Check sheet for the modelled part. Datum: model origin and axes. Units: mm. A direction names the side the tool comes from. Coordinates: 2 decimals unless noted, no trailing zeros. Write each loop counter-clockwise with the first axis right and the second up, starting at its lowest first coordinate (ties: lowest second). Pieces come first, ordered by that corner, then holes. Notation, with made-up numbers: M 49.5,-28.5 L 85.5,-28.5 A7 ccw 85.5,-24.5 Z; hole C -39,72.25 d9. An arc over 180 degrees is marked long. Answer as CSV lines item,"result". Start each with the question number.
1) Go/stop test with flat-tipped pins: pin 1 Ø3 at (y, z) = (-39.5, 29) entering from -X; pin 2 Ø3 at (x, z) = (-35.5, 78.5) entering from +Y; pin 3 Ø3 at (y, z) = (28.5, 2.5) entering from -X; pin 4 Ø12 at (x, y) = (-84.5, 26) entering from +Z. Record where each tip stops, or that it passes through.
2) Section check A-A (y = 28). Record the cut outline in (x, z) (3 decimals).
3) Material ranges on L1, parallel to Z at x = -96.5, y = -59.5 (3 decimals); L2, parallel to X at y = -33, z = 51.5 (3 decimals); L3, parallel to X at y = 55.5, z = 109, recorded low to high. Write a range as [from, to].
4) Section check B-B (x = -90). Record the cut outline in (y, z) (3 decimals).
5) Access from +Z, -Z, +X, -X, +Y, -Y to the whole of each face (thin tool, end or side, straight path). Record for faces 4 (the cylindrical face through (-64.831, -126.528, 57.817)), 5 (the flat face through (-76.2, 52, 110)), 6 (the flat face through (-9.525, 31, 58)).
6) Draft check along Z on faces 1 (the flat face through (-72, -21, 9.525)), 2 (the cylindrical face through (-107.2, -56.58, 109.6)), 3 (the flat face through (-67, -55, 0)). Enter one of: +Z half, -Z half, draft (parallel to the pull), parting line (faces both ways), or undercut.
from build123d import *

# Parameters (mm, degrees)
F1_DEPTH = 9.525
F2_DEPTH = 57.15


# Not quite as in the source:
# - ends of sketch curves that miss each other by under 0.0002 mm in the source are joined


with BuildPart() as f1:
    # F0 (on Top) → F1 (new body)
    with BuildSketch(Plane.XY):
        with BuildLine():
            Line((-9.525, -40.8894196153), (-9.525, 101.6))
            Line((-9.525, 101.6), (-76.2, 101.6))
            Line((-76.2, 101.6), (-76.2, 1.7757813176))
            ThreePointArc((-76.2, 1.7757813176), (-76.2737613091, -0.1585489984), (-76.4946168324, -2.0816447683))
            ThreePointArc((-76.4946168324, -2.0816447683), (-107.8980822653, -57.1580249287), (-168.0578880185, -77.1675992495))
            Line((-168.0578880185, -77.1675992495), (-168.0578880185, -143.8425992495))
            ThreePointArc((-168.0578880185, -143.8425992495), (-66.0749732172, -127.3460628222), (-9.525, -40.8894196153))
        make_face()
    extrude(amount=F1_DEPTH)

    # F0 (on Top) → F2 (join)
    with BuildSketch(Plane.XY):
        with BuildLine():
            ThreePointArc((-2.87076e-05, -40.8894195721), (-7.1769e-06, -40.8703254289), (0, -40.8512312749))
            Line((0, -40.8512312749), (0, 101.6))
            Line((0, 101.6), (-9.525, 101.6))
            Line((-9.525, 101.6), (-9.525, -40.8894196153))
            Line((-9.525, -40.8894196153), (-2.87076e-05, -40.8894195721))
        make_face()
        with BuildLine():
            ThreePointArc((-0.3915773599, -45.2940678749), (-0.0997672663, -43.1002807673), (-2.87076e-05, -40.8894195721))
            Line((-2.87076e-05, -40.8894195721), (-9.525, -40.8894196153))
            ThreePointArc((-9.525, -40.8894196153), (-66.0749732172, -127.3460628222), (-168.0578880185, -143.8425992495))
            Line((-168.0578880185, -143.8425992495), (-168.0578880185, -153.3675992495))
            ThreePointArc((-168.0578880185, -153.3675992495), (-60.6607327041, -135.8882486075), (-0.3915773599, -45.2940678749))
        make_face()
    extrude(amount=F2_DEPTH)

    # F3: F1 across face


with BuildPart() as f1_1:
    add(f1.part)
    add(f1.part.mirror(Plane(origin=(-44.7738585302, -61.3523725629, 57.15), x_dir=(1, 0, 0), z_dir=(0, 0, 1))))


solid = f1_1.part
Results found:
1,pin 1,"stops at x = -9.54"
1,pin 2,"stops at y = -97.6"
1,pin 3,"stops at x = -76.2"
1,pin 4,"passes through"
2,outline,"M -76.2,0 L 0,0 L 0,114.3 L -76.2,114.3 L -76.2,104.775 L -9.525,104.775 L -9.525,9.525 L -76.2,9.525 Z"
3,L1,"z = [0, 9.525], [104.775, 114.3]"
3,L2,"x = [-9.525, 0]"
3,L3,"x = [-76.2, 0]"
4,outline,"M -150.149,0 L -37.253,0 L -37.253,9.525 L -139.525,9.525 L -139.525,104.775 L -37.253,104.775 L -37.253,114.3 L -150.149,114.3 Z"
5,face 4,"+Y"
5,face 5,"+Z, -Z, -X, +Y"
5,face 6,"-X, +Y"
6,face 1,"undercut"
6,face 2,"draft"
6,face 3,"-Z half"
